Part print with two shaded views. Sizes in mm from the minimum x, y, z corner. Give positions to 0.01 mm unless a question says otherwise; leave off trailing zeros. Loops run counter-clockwise (first coordinate to the right, second up) from the corner with the lowest first, then second, coordinate; pieces in that order, holes last. Notation, with made-up numbers: M 70,60.5 L 127,60.5 A24 ccw 127,77.5 Z; hole C 13,-30.5 d2. An arc over 180 degrees is marked long. Answer as a JSON object with one key per item and string values. Group by question number.
1. Drop a flat-ended pin along its axis: pin 1 Ø5 at (x, y) = (3.415, 11.465) entering from +Z (1 decimal). Give the stop position or say it passes through.
2. Slice it at A-A (z = 0.4). List the corners of the cut face in (x, y) (1 decimal).
3. Drill centre lines: line 1 along X through (y, z) = (10.25, 1.05) (1 decimal); line 2 along X through (y, z) = (10, 1.05); line 3 along Y through (x, z) = (4.5, 0.95). Where is each one in solid material? Low to high. Write a range as [from, to].
4. Slice it at B-B (y = 10.75). Give the number of separate pieces and of enclosed holes in the cut face.
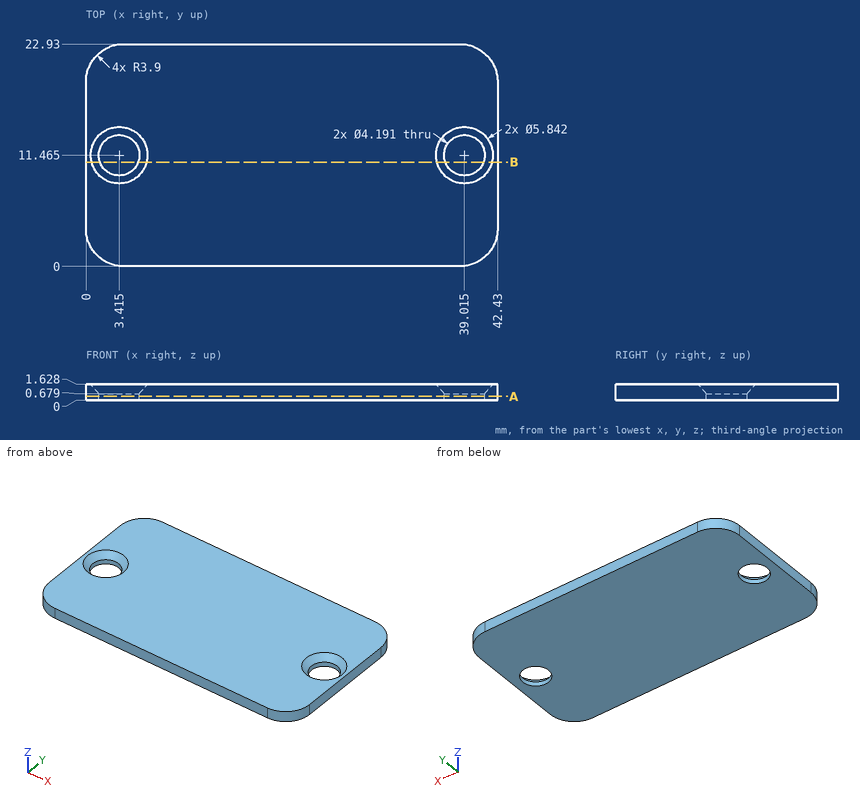
Established:
{
 "1": {"pin 1": "stops at z = 1.1"},
 "2": {"outline": "M 0,3.9 A3.9 ccw 3.9,0 L 38.5,0 A3.9 ccw 42.4,3.9 L 42.4,19 A3.9 ccw 38.5,22.9 L 3.9,22.9 A3.9 ccw 0,19 Z; hole C 3.4,11.5 d4.2; hole C 39,11.5 d4.2"},
 "3": {"line 1": "x = [0, 1.3], [5.5, 36.9], [41.1, 42.4]", "line 2": "x = [0, 1.49], [5.34, 37.09], [40.94, 42.43]", "line 3": "y = [0, 9.4], [13.53, 22.93]"},
 "4": {"separate pieces": "3", "enclosed holes": "0"}
}
